Check sheet for the modelled part. Datum: model origin and axes. Units: mm. Face numbers are marked on the shaded views. A direction names the side the tool comes from. Coordinates: 2 decimals unless noted, no trailing zeros. Write each loop counter-clockwise with the first axis right and the second up, starting at its lowest first coordinate (ties: lowest second). Pieces come first, ordered by that corner, then holes. Notation, with made-up numbers: (35, 40.5) -> (88, 40.5) arc R11 cw to (88, 47.5) -> close; hole circle Ø5 at (38, -38.75). An arc over 180 degrees is marked (long way). One line per item, written item: value. Start each with the question number.
1) Sectioned sample at A-A on y = 11. Enter the section's corners in (x, z), plus the area to 3 significant figures.
2) Draft check along Z on the marked faces 1, 2 and 3. Enter one of: +Z half, -Z half, draft (parallel to the pull), parting line (faces both ways), or undercut.
3) Scan lines: line 1 along Y through (x, z) = (0, 13.35); line 2 along X through (y, z) = (100, -17.85); line 3 along Y through (x, z) = (5.5, -9). Record each from-to range of solid material in increasing order. Write a range as [from, to].
4) Set-up check for the marked faces 4 and 5: record each of +Z, -Z, +X, -X, +Y, -Y from which the full face is reachable in a straight line by a thin tool's end or side.
5) Sectioned sample at B-B on x = 1. Give the number of separate pieces and of enclosed holes in the cut face, plus the area to 3 significant figures.
6) Gauge pin test, flat ends, axial feed: P1, Ø1.5, axis at x = 11, y = 14.5, coming from the +Z side; P2, Ø1.6, axis at y = 94, z = 14.5, coming from the +X side; P3, Ø6, axis at y = 93.5, z = -14, coming from the -X side. Record the tip position at first contact, or that the pin passes through.
```python
from build123d import *

# Parameters (mm, degrees)
CROQUIS1_R                 = 20
SALIENTE_EXTRUIR1_DEPTH    = 110
CORTAR_EXTRUIR1_DEPTH      = 110
CORTAR_EXTRUIR1_DEPTH_BACK = 110
CORTAR_EXTRUIR2_DEPTH      = 110
CORTAR_EXTRUIR2_DEPTH_BACK = 110
CROQUIS4_R                 = 4
CROQUIS5_R                 = 6
CORTAR_EXTRUIR4_DEPTH      = 4
CORTAR_EXTRUIR5_DEPTH      = 44
CHAFL_N1_SIZE              = 1


with BuildPart() as part:
    # Croquis1 → Saliente-Extruir1 (new body)
    with BuildSketch(Plane(origin=(0, 0, 0), x_dir=(1, 0, 0), z_dir=(0, 1, 0))):
        with Locations(Location((0, 0, 0), (0, 0, 270))):
            Circle(CROQUIS1_R)
    extrude(amount=SALIENTE_EXTRUIR1_DEPTH)

    # Croquis2 → Cortar-Extruir1 (cut, two sides: drawn at the far end of the back side and taken through both)
    with BuildSketch(Plane.XY.offset(-CORTAR_EXTRUIR1_DEPTH_BACK)):
        with BuildLine():
            Line((-10, 90), (-10, 100))
            ThreePointArc((-10, 100), (-7.071067812, 107.071067812), (0, 110))
            Line((0, 110), (-20, 110))
            Line((-20, 110), (-20, 75.718519933))
            Line((-20, 75.718519933), (-10, 90))
        make_face()
        with BuildLine():
            Line((20, 110), (0, 110))
            ThreePointArc((0, 110), (7.071067812, 107.071067812), (10, 100))
            Line((10, 100), (10, 90))
            Line((10, 90), (20, 75.718519933))
            Line((20, 75.718519933), (20, 110))
        make_face()
    extrude(amount=CORTAR_EXTRUIR1_DEPTH + CORTAR_EXTRUIR1_DEPTH_BACK, mode=Mode.SUBTRACT)

    # Croquis4 → Cortar-Extruir2 (cut, two sides: drawn at the far end of the back side and taken through both)
    with BuildSketch(Plane.XY.offset(-CORTAR_EXTRUIR2_DEPTH_BACK)):
        with Locations(Location((0, 100, 0), (0, 0, 180))):
            Circle(CROQUIS4_R)
    extrude(amount=CORTAR_EXTRUIR2_DEPTH + CORTAR_EXTRUIR2_DEPTH_BACK, mode=Mode.SUBTRACT)

    # Croquis3 → Cortar-Revoluci_n1 (revolve, cut)
    with BuildSketch(Plane(origin=(0, 0, 0), x_dir=(0, 0, -1), z_dir=(1, 0, 0))):
        with BuildLine():
            Line((-12, 110), (12, 110))
            Line((12, 110), (12, 84))
            ThreePointArc((12, 84), (0, 72), (-12, 84))
            Line((-12, 84), (-12, 110))
        make_face()
    revolve(axis=Axis((0, 110, 12), (0, 0, -1)), mode=Mode.SUBTRACT)

    # Croquis5 → Cortar-Extruir4 (cut)
    with BuildSketch(Plane.XY.offset(20)):
        with Locations((0, 100)):
            Circle(CROQUIS5_R)
    cortar_extruir4 = extrude(amount=-CORTAR_EXTRUIR4_DEPTH, mode=Mode.SUBTRACT)

    # Simetr_a1: Cortar-Extruir4 across plane
    add(cortar_extruir4.mirror(Plane.XY), mode=Mode.SUBTRACT)

    # Croquis6 → Cortar-Revoluci_n2 (revolve, cut)
    with BuildSketch(Plane.XY, mode=Mode.PRIVATE) as cortar_revoluci_n2_sk:
        Polygon((-9, 0), (0, 0), (0, 70), (-14, 70), (-14, 30), (-9, 30), align=None)
    revolve(cortar_revoluci_n2_sk.sketch.rotate(Axis((0, 70, 0), (0, -1, 0)), 270), axis=Axis((0, 70, 0), (0, -1, 0)), mode=Mode.SUBTRACT)

    # Croquis7 → Cortar-Extruir5 (cut)
    with BuildSketch(Plane.XZ):
        with BuildLine():
            Line((-9.239334584, 3.827057692), (-8.314915793, 3.444150891))
            ThreePointArc((-8.314915793, 3.444150891), (-9, 0), (-8.314915793, -3.444150891))
            Line((-8.314915793, -3.444150891), (-9.239334584, -3.827057692))
            ThreePointArc((-9.239334584, -3.827057692), (-7.071480543, -7.071480543), (-3.827057692, -9.239334584))
            Line((-3.827057692, -9.239334584), (-3.444150891, -8.314915793))
            ThreePointArc((-3.444150891, -8.314915793), (0, -9), (3.444150891, -8.314915793))
            Line((3.444150891, -8.314915793), (3.827057692, -9.239334584))
            ThreePointArc((3.827057692, -9.239334584), (7.071480543, -7.071480543), (9.239334584, -3.827057692))
            Line((9.239334584, -3.827057692), (8.314915793, -3.444150891))
            ThreePointArc((8.314915793, -3.444150891), (9, 0), (8.314915793, 3.444150891))
            Line((8.314915793, 3.444150891), (9.239334584, 3.827057692))
            ThreePointArc((9.239334584, 3.827057692), (7.071480543, 7.071480543), (3.827057692, 9.239334584))
            Line((3.827057692, 9.239334584), (3.444150891, 8.314915793))
            ThreePointArc((3.444150891, 8.314915793), (0, 9), (-3.444150891, 8.314915793))
            Line((-3.444150891, 8.314915793), (-3.827057692, 9.239334584))
            ThreePointArc((-3.827057692, 9.239334584), (-7.071480543, 7.071480543), (-9.239334584, 3.827057692))
        make_face()
    extrude(amount=-CORTAR_EXTRUIR5_DEPTH, mode=Mode.SUBTRACT)

    # Chafl_n1
    chafl_n1_edges = [part.edges().sort_by_distance(p)[0] for p in [
        (0, 0, -20),
    ]]
    chamfer(chafl_n1_edges, length=CHAFL_N1_SIZE)


solid = part.part
```
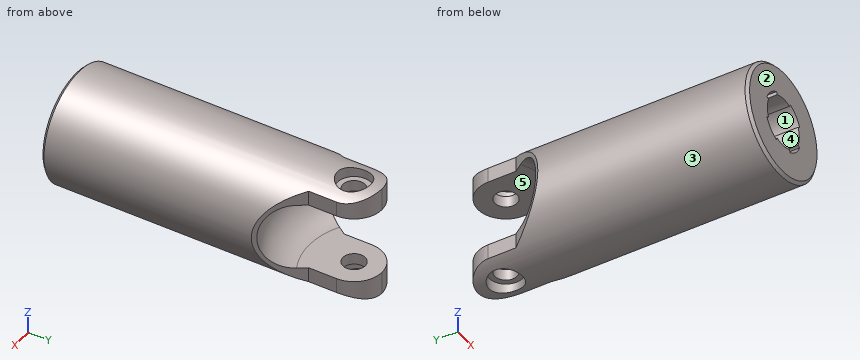
Answers:
1. outline: circle Ø40 at (0, 0); hole (-9.24, -3.83) arc R10 ccw to (-3.83, -9.24) -> (-3.44, -8.31) arc R9 ccw to (3.44, -8.31) -> (3.83, -9.24) arc R10 ccw to (9.24, -3.83) -> (8.31, -3.44) arc R9 ccw to (8.31, 3.44) -> (9.24, 3.83) arc R10 ccw to (3.83, 9.24) -> (3.44, 8.31) arc R9 ccw to (-3.44, 8.31) -> (-3.83, 9.24) arc R10 ccw to (-9.24, 3.83) -> (-8.31, 3.44) arc R9 ccw to (-8.31, -3.44) -> close
1. area: 972 mm2
2. face 1: undercut
2. face 2: draft
2. face 3: parting line
3. line 1: y = [0, 30], [70, 96], [104, 110]
3. line 2: x = [-9.02, -6], [6, 9.02]
3. line 3: y = [0, 30], [70, 76.51]
4. face 4: -Y
4. face 5: +Y
5. separate pieces: 3
5. enclosed holes: 0
5. area: 1,730 mm2
6. P1: stops at z = 17.17
6. P2: stops at x = 10
6. P3: stops at x = -10
